Could you check a few things on this model? Use its own coordinates, in mm. A direction names the side the tool comes from. Coordinates: 2 decimals unless noted, no trailing zeros. Loops run counter-clockwise (first coordinate to the right, second up) from the corner with the lowest first, then second, coordinate; pieces in that order, holes last. Notation, with made-up numbers: (58.5, 67) - (97.5, 67) arc R22 ccw to (97.5, 101) - close; hole circle Ø3 at (-35.75, -24). An arc over 180 degrees is marked (long way). One line per item, written item: value. Start each with the question number.
(1) On a 3-axis mill with a long thin cutter (end or side, diameter ignored), from which of +Z, -Z, +X, -X, +Y, -Y can I reach the whole of each face in a straight line? I mean faces 1 (the face through (11, 11, -2)), 2 (the face through (-17, 23, 1)), 3 (the face through (17, 23, 1)), 4 (the face through (23, -17, 1)). Say none if no direction works.
(2) If we mould it in two halves opening along Y, with no side actions, what happens to faces 5 (the face through (-18.09, -17.54, 0.46)), 6 (the face through (-24.901, 0, 0)), 7 (the face through (19.131, 19.192, 0.535))? For each: pulls with the +Y half, pulls with the -Y half, needs draft (parallel to the pull), parting line crosses it, or undercut.
(3) If I drill on line 1 along Y through (x, z) = (-16.9, 1.85); line 2 along Y through (x, z) = (-21.5, 1); line 3 along X through (y, z) = (6.5, 0.75), over which ranges is the centre line in solid material (lowest first)? Write a range as from..to.
(4) If we section it at C-C on z = -4.25: Write out the boundary of the cut face in (x, y), then the cut area to 3 significant figures.
(5) If we section it at B-B on x = -2.5: Write out the boundary of the cut face in (y, z).
(6) I'm going to push flat-ended pins straight in: P1, Ø1.8, axis at y = -23, z = -0.5, coming from the -X side; P2, Ø3, axis at x = 23.5, z = 1, coming from the +Y side; P3, Ø3, axis at x = -5, y = -5.5, coming from the +Z side; P4, Ø6, axis at y = -12.5, z = -4, coming from the -X side. Where does each tip first touch, or does it pass through?
(7) If we section it at A-A on y = 13: Write out the boundary of the cut face in (x, z), then the cut area to 3 significant figures.
Autodesk Inventor part; units mm, degrees
ref_plane "YZ Plane" through (0, 0, 0) normal (1, 0, 0) x (0, 1, 0)
ref_plane "XZ Plane" through (0, 0, 0) normal (0, 1, 0) x (-1, 0, 0)
ref_plane "XY Plane" through (0, 0, 0) normal (0, 0, 1) x (1, 0, 0)
sketch "Sketch1" plane through (0, 0, 0) normal (0, 0, 1) x (1, 0, 0)
  line L0 (-38.8739, 0) -> (58.9391, 0) construction
  line L1 (0, -36.2399) -> (0, 43.1348) construction
  line L2 (0, 0) -> (31.7956, 31.7956) construction
  line L3 (0, 0) -> (44.9658, 0) construction
  line L4 (0, 24.9006) -> (16.8, 24.9006)
  line L5 (16.8, 24.9006) -> (16.8, 21.2406)
  line L6 (16.8, 21.2406) -> (19.0203, 19.0203)
  line L7 (24.9006, 0) -> (24.9006, 16.8)
  line L8 (24.9006, 16.8) -> (21.2406, 16.8)
  line L9 (21.2406, 16.8) -> (19.0203, 19.0203)
  line L10 (0, 24.9006) -> (-16.8, 24.9006)
  line L11 (-16.8, 24.9006) -> (-16.8, 21.2406)
  line L12 (-16.8, 21.2406) -> (-19.0203, 19.0203)
  line L13 (-24.9006, 0) -> (-24.9006, 16.8)
  line L14 (-24.9006, 16.8) -> (-21.2406, 16.8)
  line L15 (-21.2406, 16.8) -> (-19.0203, 19.0203)
  line L16 (0, -24.9006) -> (16.8, -24.9006)
  line L17 (16.8, -24.9006) -> (16.8, -21.2406)
  line L18 (16.8, -21.2406) -> (19.0203, -19.0203)
  line L19 (24.9006, 0) -> (24.9006, -16.8)
  line L20 (24.9006, -16.8) -> (21.2406, -16.8)
  line L21 (21.2406, -16.8) -> (19.0203, -19.0203)
  line L22 (0, -24.9006) -> (-16.8, -24.9006)
  line L23 (-16.8, -24.9006) -> (-16.8, -21.2406)
  line L24 (-16.8, -21.2406) -> (-19.0203, -19.0203)
  line L25 (-24.9006, 0) -> (-24.9006, -16.8)
  line L26 (-24.9006, -16.8) -> (-21.2406, -16.8)
  line L27 (-21.2406, -16.8) -> (-19.0203, -19.0203)
  circle A0 centre (0, 0) radius 13.675
  dimension "d0" = 45
  dimension "d1" = 16.8
  dimension "d2" = 3.66
  dimension "d3" = 3.14
  dimension "d4" = 27.35
extrude "Extrusion1" add sketch "Sketch1" along normal blind 3
sketch "Sketch2" plane through (0, 0, 3) normal (0, 0, 1) x (1, 0, 0)
  circle A0 centre (0, 0) radius 13.675 construction
  line L0 (16.8, 24.9006) -> (-16.8, 24.9006) construction
  line L1 (-16.8, 24.9006) -> (-16.8, 21.2406) construction
  line L2 (-16.8, 21.2406) -> (-21.2406, 16.8) construction
  line L3 (-21.2406, 16.8) -> (-24.9006, 16.8) construction
  line L4 (-24.9006, 16.8) -> (-24.9006, -16.8) construction
  line L5 (-24.9006, -16.8) -> (-21.2406, -16.8) construction
  line L6 (-21.2406, -16.8) -> (-16.8, -21.2406) construction
  line L7 (-16.8, -21.2406) -> (-16.8, -24.9006) construction
  line L8 (-16.8, -24.9006) -> (16.8, -24.9006) construction
  line L9 (16.8, -24.9006) -> (16.8, -21.2406) construction
  line L10 (16.8, -21.2406) -> (21.2406, -16.8) construction
  line L11 (21.2406, -16.8) -> (24.9006, -16.8) construction
  line L12 (24.9006, -16.8) -> (24.9006, 16.8) construction
  line L13 (24.9006, 16.8) -> (21.2406, 16.8) construction
  line L14 (21.2406, 16.8) -> (16.8, 21.2406) construction
  line L15 (16.8, 21.2406) -> (16.8, 24.9006) construction
  line L16 (-34.8609, 0) -> (34.8609, 0) construction
  line L17 (0, -34.8609) -> (0, 34.8609) construction
  circle A1 centre (13, -13) radius 2.5
  circle A2 centre (-13, -13) radius 2.5
  dimension "d7" = 5
  dimension "d8" = 13
  dimension "d9" = 13
extrude "Extrusion2" [suppressed]
sketch "Sketch3" plane through (0, 0, 0) normal (1, 0, 0) x (0, 1, 0)
  line L0 (-13.675, 3) -> (13.675, 3) construction
  line L1 (24.9006, 3) -> (21.2406, 3) construction
  line L2 (21.2406, 3) -> (16.8, 3) construction
  line L3 (16.8, 3) -> (-16.8, 3) construction
  line L4 (-16.8, 3) -> (-21.2406, 3) construction
  line L5 (-21.2406, 3) -> (-24.9006, 3) construction
  line L6 (-24.9006, 3) -> (-21.2406, 3) construction
  line L7 (-21.2406, 3) -> (-16.8, 3) construction
  line L8 (-16.8, 3) -> (16.8, 3) construction
  line L9 (16.8, 3) -> (21.2406, 3) construction
  line L10 (21.2406, 3) -> (24.9006, 3) construction
  line L11 (24.9006, 0) -> (21.2406, 0) construction
  line L12 (24.9006, 0) -> (24.9006, 3) construction
  line L13 (21.2406, 3) -> (24.9006, 3) construction
  line L14 (21.2406, 0) -> (21.2406, 3) construction
  line L15 (21.2406, 0) -> (16.8, 0) construction
  line L16 (21.2406, 0) -> (21.2406, 3) construction
  line L17 (16.8, 3) -> (21.2406, 3) construction
  line L18 (16.8, 0) -> (16.8, 3) construction
  line L19 (16.8, 0) -> (-16.8, 0) construction
  line L20 (16.8, 0) -> (16.8, 3) construction
  line L21 (-16.8, 3) -> (16.8, 3) construction
  line L22 (-16.8, 0) -> (-16.8, 3) construction
  line L23 (-16.8, 0) -> (-21.2406, 0) construction
  line L24 (-16.8, 0) -> (-16.8, 3) construction
  line L25 (-21.2406, 3) -> (-16.8, 3) construction
  line L26 (-21.2406, 0) -> (-21.2406, 3) construction
  line L27 (-21.2406, 0) -> (-24.9006, 0) construction
  line L28 (-21.2406, 0) -> (-21.2406, 3) construction
  line L29 (-24.9006, 3) -> (-21.2406, 3) construction
  line L30 (-24.9006, 0) -> (-24.9006, 3) construction
  line L31 (-13.675, 3) -> (13.675, 3) construction
  line L32 (13.675, 0) -> (-13.675, 0) construction
  line L33 (16.8, 3) -> (-16.8, 3)
  arc A0 (0, -10.675) -> (13.675, 3) centre (0, 3) ccw
  line L34 (0, -20.1765) -> (0, 6.8627) construction
  arc A1 (0, -12.675) -> (15.675, 3) centre (0, 3) ccw
  line L35 (0, -10.675) -> (0, -12.675)
  line L36 (15.675, 3) -> (13.675, 3)
revolve "Revolution1" add sketch "Sketch3" angle 360 about axis through (0, 0, -10) along (0, 0, 1)
sketch "Skizze4" plane through (0, 0, 3) normal (0, 0, 1) x (1, 0, 0)
  circle A0 centre (0, 0) radius 13.675 construction
  line L0 (16.8, 24.9006) -> (-16.8, 24.9006) construction
  line L1 (-16.8, 24.9006) -> (-16.8, 21.2406)
  line L2 (-16.8, 21.2406) -> (-21.2406, 16.8)
  line L3 (-21.2406, 16.8) -> (-24.9006, 16.8)
  line L4 (-24.9006, 16.8) -> (-24.9006, -16.8) construction
  line L5 (-24.9006, -16.8) -> (-21.2406, -16.8)
  line L6 (-21.2406, -16.8) -> (-16.8, -21.2406)
  line L7 (-16.8, -21.2406) -> (-16.8, -24.9006)
  line L8 (-16.8, -24.9006) -> (16.8, -24.9006) construction
  line L9 (16.8, -24.9006) -> (16.8, -21.2406)
  line L10 (16.8, -21.2406) -> (21.2406, -16.8)
  line L11 (21.2406, -16.8) -> (24.9006, -16.8)
  line L12 (24.9006, -16.8) -> (24.9006, 16.8) construction
  line L13 (24.9006, 16.8) -> (21.2406, 16.8)
  line L14 (21.2406, 16.8) -> (16.8, 21.2406)
  line L15 (16.8, 21.2406) -> (16.8, 24.9006)
  line L16 (-17, 25.1006) -> (17, 25.1006) construction
  line L17 (17, 25.1006) -> (17, 21.3235)
  line L18 (17, 21.3235) -> (21.3235, 17)
  line L19 (21.3235, 17) -> (25.1006, 17)
  line L20 (25.1006, 17) -> (25.1006, -17) construction
  line L21 (25.1006, -17) -> (21.3235, -17)
  line L22 (21.3235, -17) -> (17, -21.3235)
  line L23 (17, -21.3235) -> (17, -25.1006)
  line L24 (17, -25.1006) -> (-17, -25.1006) construction
  line L25 (-17, -25.1006) -> (-17, -21.3235)
  line L26 (-17, -21.3235) -> (-21.3235, -17)
  line L27 (-21.3235, -17) -> (-25.1006, -17)
  line L28 (-25.1006, -17) -> (-25.1006, 17) construction
  line L29 (-25.1006, 17) -> (-21.3235, 17)
  line L30 (-21.3235, 17) -> (-17, 21.3235)
  line L31 (-17, 21.3235) -> (-17, 25.1006)
  line L32 (-24.9006, 16.8) -> (-24.9006, 17)
  line L33 (16.8, 24.9006) -> (-16.8, 24.9006)
  line L34 (-16.8, 24.9006) -> (-17, 24.9006)
  line L35 (16.8, 24.9006) -> (17, 24.9006)
  line L36 (24.9006, -16.8) -> (24.9006, 16.8)
  line L37 (24.9006, 16.8) -> (24.9006, 17)
  line L38 (24.9006, -16.8) -> (24.9006, -17)
  line L39 (16.8, -24.9006) -> (16.8, -21.2406)
  line L40 (16.8, -24.9006) -> (17, -24.9006)
  line L41 (-16.8, -24.9006) -> (-17, -24.9006)
  line L42 (-24.9006, -16.8) -> (-24.9006, 16.8)
  line L43 (-24.9006, -16.8) -> (-24.9006, -17)
  dimension "d15" = 0.2
extrude "IM_offset" add sketch "Skizze4" against normal up to surface (3 mm away)
sketch "Sketch6" plane through (0, 0, 3) normal (0, 0, 1) x (1, 0, 0)
  circle A0 centre (-16.9, -16.9) radius 1.35
  circle A1 centre (16.8404, -16.8404) radius 1.35
  point P0 (0, 0)
hole "Hole1" at (-16.9, -16.9, 3) at (16.8404, -16.8404, 3) direction (0, 0, -1) diameter 2.7 end through all
sketch "Sketch7" plane through (0, 0, 0) normal (0, 0, -1) x (-1, 0, 0)
  circle A0 centre (16.9, -16.9) radius 1.35
  circle A1 centre (-16.8404, -16.8404) radius 1.35
  circle A2 centre (0, 0) radius 15.3852
  line L0 (17, 24.9006) -> (-17, 24.9006)
  line L1 (-17, 24.9006) -> (-17, 21.3235)
  line L2 (-17, 21.3235) -> (-21.3235, 17)
  line L3 (-21.3235, 17) -> (-24.9006, 17)
  line L4 (-24.9006, 17) -> (-24.9006, -17)
  line L5 (-24.9006, -17) -> (-21.3235, -17)
  line L6 (-21.3235, -17) -> (-17, -21.3235)
  line L7 (-17, -21.3235) -> (-17, -24.9006)
  line L8 (-17, -24.9006) -> (17, -24.9006)
  line L9 (17, -24.9006) -> (17, -21.3235)
  line L10 (17, -21.3235) -> (21.3235, -17)
  line L11 (21.3235, -17) -> (24.9006, -17)
  line L12 (24.9006, -17) -> (24.9006, 17)
  line L13 (24.9006, 17) -> (21.3235, 17)
  line L14 (21.3235, 17) -> (17, 21.3235)
  line L15 (17, 21.3235) -> (17, 24.9006)
  circle A3 centre (0, 0) radius 13.675
extrude "Extrusion4" add sketch "Sketch7" along normal blind 2 contours A2 | L15 L14 L13 L12 L11 L10 L9 L8 L7 L6 L5 L4 L3 L2 L1 L0
equation "\"d9\" = d8"
properties part number "20_Cube_Insert_Eye_v3"
Values:
1. face 1: -Z
1. face 2: +Z, -Z, -X, +Y
1. face 3: +Z, -Z, +X, +Y
1. face 4: +Z, -Z, +X, -Y
2. face 5: undercut
2. face 6: needs draft
2. face 7: pulls with the +Y half
3. line 1: y = -24.9..-18.25, -15.55..24.9
3. line 2: y = -17..17
3. line 3: x = -24.9..-11.82, 11.82..24.9
4. outline: circle Ø27.8 at (0, 0); hole circle Ø23.19 at (0, 0)
4. area: 184 mm2
5. outline: (-24.9, -2) - (-14.64, -2) arc R15.47 ccw to (14.64, -2) - (24.9, -2) - (24.9, 3) - (13.44, 3) arc R13.44 cw to (-13.44, 3) - (-24.9, 3) - close
6. P1: stops at x = -17
6. P2: stops at y = 17
6. P3: stops at z = -7.35
6. P4: stops at x = -24.9
7. outline: (-24.9, -2) - (-7.19, -2) arc R8.76 ccw to (7.19, -2) - (24.9, -2) - (24.9, 3) - (4.24, 3) arc R4.24 cw to (-4.24, 3) - (-24.9, 3) - close
7. area: 259 mm2
